Here's how the part is built. I have some questions about the finished solid (model axes, mm). Face numbers are marked on the shaded views. A direction names the side the tool comes from. Coordinates: 2 decimals unless noted, no trailing zeros. Loops run counter-clockwise (first coordinate to the right, second up) from the corner with the lowest first, then second, coordinate; pieces in that order, holes last. Notation, with made-up numbers: (85.25, 85.25) - (113.25, 85.25) arc R19 cw to (113.25, 100.25) - close; hole circle Ø9 at (-5, 9.25). An arc over 180 degrees is marked (long way). Use a Markdown table: item, result.
Autodesk Inventor part; units mm, degrees
ref_plane "YZ Plane" through (0, 0, 0) normal (1, 0, 0) x (0, 1, 0)
ref_plane "XZ Plane" through (0, 0, 0) normal (0, 1, 0) x (-1, 0, 0)
ref_plane "XY Plane" through (0, 0, 0) normal (0, 0, 1) x (1, 0, 0)
sketch "Sketch1" plane through (0, 0, 0) normal (0, 0, 1) x (1, 0, 0)
  line L0 (-6.635, 1.85) -> (6.635, 1.85)
  line L1 (6.635, 1.85) -> (6.635, -1.85)
  line L2 (6.635, -1.85) -> (0.7071, -1.85)
  line L3 (-6.635, -1.85) -> (-6.635, 1.85)
  line L4 (-6.635, 1.85) -> (6.635, -1.85) construction
  line L5 (6.635, 1.85) -> (-6.635, -1.85) construction
  line L6 (-6.635, 0.85) -> (-4.035, 0.85)
  line L7 (-4.035, 0.85) -> (-4.035, -0.85)
  line L8 (-4.035, -0.85) -> (-6.635, -0.85)
  line L9 (-6.635, -0.85) -> (-6.635, 0.85)
  line L10 (6.635, 0.85) -> (4.035, 0.85)
  line L11 (4.035, 0.85) -> (4.035, -0.85)
  line L12 (4.035, -0.85) -> (6.635, -0.85)
  line L13 (6.635, -0.85) -> (6.635, 0.85)
  line L14 (-4.035, 0) -> (-6.635, 0) construction
  line L15 (6.635, 0) -> (4.035, 0) construction
  circle A0 centre (0, -1.6) radius 0.75
  line L16 (-0.75, -2.35) -> (0.75, -2.35)
  line L17 (0.75, -2.35) -> (0.75, -1.85)
  line L18 (-0.75, -2.35) -> (-0.75, -1.85)
  line L19 (-0.7071, -1.85) -> (-6.635, -1.85)
  line L20 (0.7071, -1.85) -> (-0.7071, -1.85)
  line L21 (-6.635, -1.85) -> (-0.75, -3.35)
  line L22 (-0.75, -3.35) -> (0.75, -3.35)
  line L23 (0.75, -3.35) -> (6.635, -1.85)
  line L24 (-0.75, -1.85) -> (-0.75, -1.6)
  line L25 (0.75, -1.85) -> (0.75, -1.6)
  point P0 (0, 0)
  point P1 (0, 0)
  point P2 (0, 0)
  dimension "d0" = 2.6
  dimension "d1" = 2.6
  dimension "d2" = 13.27
  dimension "d3" = 1.7
  dimension "d4" = 1
  dimension "d7" = 1.5
  dimension "d8" = 1
extrude "Extrusion2" add sketch "Sketch1" along normal blind 6 contours L0 L1 L10 L11 L12 L2 L25 A0 L24 L19 L3 L8 L7 L6 | L19 L18 L16 L17 L2 L23 L22 L21
chamfer "Chamfer1" distance 0.7 angle 45 2 edges at (-4.035, 0, 6) (4.035, 0, 6)
equation "\"d1\" = d0"
properties part number "glass_holder"
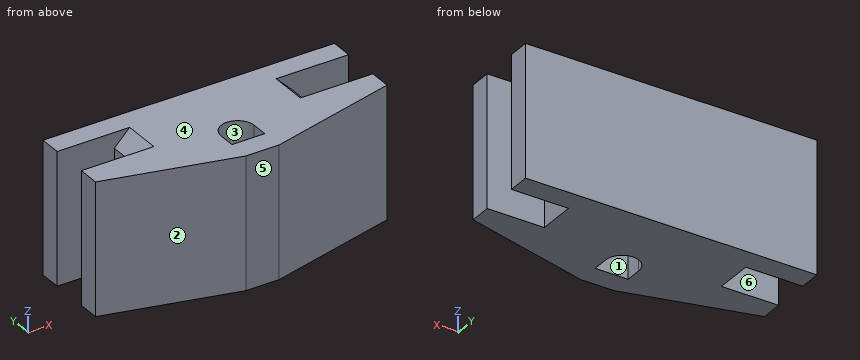
Q1. Which directions (+Z, -Z, +X, -X, +Y, -Y) give clear straight access to the entire face, cutting with the end or side of a thin tool? Please do the marked faces 1 and 2.
Check values:
| item | result |
|---|---|
| face 1 | +Z, -Z |
| face 2 | +Z, -Z, -X, -Y |
Q2. I want a section at A-A, the plane x = 0. Write out the boundary of the cut face in (y, z), then the cut area to 3 significant figures.
Check values:
| item | result |
|---|---|
| outline | (-3.35, 0) - (-2.35, 0) - (-2.35, 6) - (-3.35, 6) - close; (-0.85, 0) - (1.85, 0) - (1.85, 6) - (-0.85, 6) - close |
| area | 22.2 mm^2 |
Q3. I want a section at D-D, the plane y = -0.5. Write out the boundary of the cut face in (x, z) (3 decimals), then the cut area to 3 significant figures.
Check values:
| item | result |
|---|---|
| outline | (-4.035, 0) - (4.035, 0) - (4.035, 5.3) - (3.335, 6) - (-3.335, 6) - (-4.035, 5.3) - close |
| area | 47.9 mm^2 |
Q4. Please list where these lines run through material, in increasing order: L1, parallel to X at y = -1.7, z = 2.75 (3 decimals); L2, parallel to Y at x = 5.75, z = 4.5. Write a range as from..to.
Check values:
| item | result |
|---|---|
| L1 | -6.635..-0.75, 0.75..6.635 |
| L2 | -2.08..-0.85, 0.85..1.85 |
Q5. Will these pins go through, and if not, where does the flat tip stop? P1, Ø0.5, axis at y = 0.5, z = 4, coming from the +X side (3 decimals); P2, Ø1.4, axis at y = 0, z = 4, coming from the -X side (3 decimals); P3, Ø1.6, axis at x = -5.5, z = 4.5, coming from the -Y side.
Check values:
| item | result |
|---|---|
| P1 | x = 4.035 |
| P2 | x = -4.035 |
| P3 | y = -2.34 |
Q6. I want a section at C-C, the plane y = -1.1. Write out the boundary of the cut face in (x, z) (3 decimals), then the cut area to 3 significant figures.
Check values:
| item | result |
|---|---|
| outline | (-6.635, 0) - (-0.559, 0) - (-0.559, 6) - (-6.635, 6) - close; (0.559, 0) - (6.635, 0) - (6.635, 6) - (0.559, 6) - close |
| area | 72.9 mm^2 |
Q7. If we mould it in two halves opening along Y, with no side actions, what happens to the marked faces 3, 4, 5 and 6? For each: pulls with the +Y half, pulls with the -Y half, needs draft (parallel to the pull), parting line crosses it, or undercut.
Check values:
| item | result |
|---|---|
| face 3 | undercut |
| face 4 | needs draft |
| face 5 | pulls with the -Y half |
| face 6 | undercut |
Q8. I want a section at B-B, the plane z = 4.65. Write out the boundary of the cut face in (x, y) (3 decimals).
Check values:
| item | result |
|---|---|
| outline | (-6.635, -1.85) - (-0.75, -3.35) - (0.75, -3.35) - (6.635, -1.85) - (6.635, -0.85) - (4.035, -0.85) - (4.035, 0.85) - (6.635, 0.85) - (6.635, 1.85) - (-6.635, 1.85) - (-6.635, 0.85) - (-4.035, 0.85) - (-4.035, -0.85) - (-6.635, -0.85) - close; hole (-0.75, -2.35) - (0.75, -2.35) - (0.75, -1.6) arc R0.75 ccw to (-0.75, -1.6) - close |
